Model file for the job. Use its own axes, mm. Face numbers are marked on the shaded views. A direction names the side the tool comes from. Coordinates: 2 decimals unless noted, no trailing zeros. Order: outer loops, then holes, each group sorted by start corner. A loop starts at its lowest first (then second) coordinate and runs counter-clockwise, first axis right, second up. Notation, with made-up numbers: (-30.5, 41) -> (7.5, 41) arc R29 ccw to (7.5, 74) -> close; hole circle Ø6 at (9, -8). An arc over 180 degrees is marked (long way). Use CSV: the item, a comma, the result in double quotes. Start each with the question number.
(1) Cut at B-B on x = 27.85. Write the cut outline in (y, z).
(2) Cut at A-A on z = 0. Write the cut outline in (x, y).
(3) Tool access for the marked faces 4, 5 and 6: list every direction of +Z, -Z, +X, -X, +Y, -Y with a clear straight run to the whole face (end or side of a thin tool).
(4) Pin check, flat tips, straight feed: pin 1 Ø3 at (y, z) = (2.5, 1.5) entering from +X; pin 2 Ø1.2 at (y, z) = (3, -11) entering from -X; pin 3 Ø4.5 at (x, z) = (13, -13) entering from +Y; pin 4 Ø8.5 at (x, y) = (27.85, -14) entering from -Z. Stop position of each tip, or through.
(5) Cut at C-C on x = 0. Write the cut outline in (y, z).
(6) Cut at D-D on y = -22. Write the cut outline in (x, z).
(7) Pull direction Z, two halves, no side cores. Call the marked faces 1, 2 and 3: pulls with the +Z half, pulls with the -Z half, needs draft (parallel to the pull), parting line crosses it, or undercut.
(8) Probe L1, parallel to X at y = 2, z = -13; L2, parallel to Z at x = 6.5, y = -8; L3, parallel to Z at x = 16.5, y = -1. List the from-to ranges inside material, lowest first.
Autodesk Inventor part; units mm, degrees
ref_plane "YZ Plane" through (0, 0, 0) normal (1, 0, 0) x (0, 1, 0)
ref_plane "XZ Plane" through (0, 0, 0) normal (0, 1, 0) x (-1, 0, 0)
ref_plane "XY Plane" through (0, 0, 0) normal (0, 0, 1) x (1, 0, 0)
sketch "Boceto1" plane through (0, 0, 0) normal (0, 1, 0) x (-1, 0, 0)
  line L0 (-17.55, 17.55) -> (17.55, 17.55)
  line L1 (17.55, 17.55) -> (17.55, -17.55)
  line L2 (17.55, -17.55) -> (-17.55, -17.55)
  line L3 (-17.55, -17.55) -> (-17.55, 17.55)
  line L4 (-17.55, 17.55) -> (17.55, -17.55) construction
  line L5 (17.55, 17.55) -> (-17.55, -17.55) construction
  circle A0 centre (0, 0) radius 11.2
  point P0 (0, 0)
  dimension "d0" = 35.1
  dimension "d1" = 35.1
  dimension "d2" = 22.4
extrude "Extrusión1" add sketch "Boceto1" along normal blind 4
sketch "Boceto2" plane through (0, 4, 0) normal (0, 1, 0) x (1, 0, 0)
  circle A0 centre (-13, -13) radius 1.7
  line L0 (13, -13) -> (-13, -13)
  line L1 (-13, -13) -> (-13, 13)
  line L2 (-13, 13) -> (13, 13)
  line L3 (13, 13) -> (13, -13)
  line L4 (13, -13) -> (-13, 13) construction
  line L5 (-13, -13) -> (13, 13) construction
  point P0 (0, 0)
  dimension "d5" = 26
  dimension "d6" = 26
  dimension "d7" = 3.4
extrude "Extrusión2" cut sketch "Boceto2" against normal through all contours L0 L1 A0 | A0 L1 L0
pattern_circular "Patrón circular1" count 4 over 360 about axis through (0, 0, 0) along (0, 1, 0) of "Extrusión2"
sketch "Boceto13" plane through (0, 4, 0) normal (0, 1, 0) x (1, 0, 0)
  line L0 (-17.55, -17.55) -> (17.55, -17.55)
  line L1 (17.55, -17.55) -> (37.85, -17.55)
  line L2 (37.85, -17.55) -> (37.85, 17.55)
  line L3 (37.85, 17.55) -> (17.55, 17.55)
  line L4 (17.55, 17.55) -> (17.55, -17.55)
  line L5 (17.55, 17.55) -> (-17.55, 17.55)
  line L6 (41.5, -10.15) -> (21.2, -10.15)
  line L7 (21.2, -10.15) -> (21.2, 10.15)
  line L8 (21.2, 10.15) -> (41.5, 10.15)
  line L9 (41.5, 10.15) -> (41.5, -10.15)
  line L10 (41.5, -10.15) -> (21.2, 10.15) construction
  line L11 (21.2, -10.15) -> (41.5, 10.15) construction
  circle A0 centre (27.85, 0) radius 2.7
  point P0 (0, 0)
  point P1 (31.35, 0)
  dimension "d43" = 20.3
  dimension "d44" = 20.3
  dimension "d45" = 20.3
  dimension "d61" = 5.4
  dimension "d62" = 10
extrude "Extrusión8" add sketch "Boceto13" against normal blind 33 contours L4 L3 L2 L8 L7 L6 L1 | L6 L7 L8 L2
sketch "Boceto14" plane through (0, -29, 0) normal (0, -1, 0) x (1, 0, 0)
  line L0 (17.55, 17.55) -> (17.55, -17.55)
  line L1 (37.85, -10.15) -> (17.55, -10.15)
  line L2 (17.55, -10.15) -> (17.55, 10.15)
  line L3 (17.55, 10.15) -> (37.85, 10.15)
  line L4 (37.85, 10.15) -> (37.85, -10.15)
  line L5 (37.85, -10.15) -> (17.55, 10.15) construction
  line L6 (17.55, -10.15) -> (37.85, 10.15) construction
  line L7 (37.85, -17.55) -> (37.85, 17.55)
  circle A0 centre (27.85, 0) radius 2.7
  point P0 (0, 0)
  point P1 (27.7, 0)
  point P2 (17.55, -10.15)
  point P3 (27.7, 0)
  dimension "d49" = 20.3
extrude "Extrusión9" cut sketch "Boceto14" against normal up to surface (29 mm away) contours L3 L4 L1 L0 | A0
sketch "Boceto15" plane through (-17.55, 0, -17.55) normal (0, 0, -1) x (-1, 0, 0)
  line L0 (-35.1, 0) -> (0, 0)
  line L1 (0, 0) -> (0, 4)
  line L2 (-55.4, 4) -> (0, 4)
  line L3 (-55.4, 4) -> (-55.4, -29)
  line L4 (-35.1, -29) -> (-55.4, -29)
  line L5 (-35.1, 0) -> (-35.1, -29)
  line L6 (0, 0) -> (0, 4)
  line L7 (-35.1, -29) -> (-55.4, -29)
  line L8 (0, 0) -> (-35.1, -29)
  point P0 (-17.55, 0)
extrude "Extrusión10" add sketch "Boceto15" along normal blind 2
mirror "Simetría1" about plane through (0, 0, 0) normal (0, 0, 1) of "Extrusión10"
sketch "Boceto16" plane through (-17.55, 0, -19.55) normal (0, 0, -1) x (-1, 0, 0)
  circle A0 centre (-45.4, -14) radius 2.7
  line L0 (-55.4, 4) -> (-55.4, -29)
  line L1 (-55.4, -29) -> (-35.1, -29)
  point P0 (-17.55, 0)
  dimension "d54" = 10
  dimension "d55" = 5.4
  dimension "d57" = 15
extrude "Extrusión11" cut sketch "Boceto16" against normal through all
fillet "Empalme1" radius 2 1 edges at (37.85, -29, -14.85)
sketch "Boceto17" plane through (-17.55, 0, -19.55) normal (0, 0, -1) x (-1, 0, 0)
  circle A0 centre (-45.4, -14) radius 2.7
  circle A1 centre (-45.4, -14) radius 4.65
  point P0 (-17.55, 0)
  dimension "d63" = 9.3
extrude "Extrusión12" cut sketch "Boceto17" against normal blind 2 contours A0 | A1
sketch "Boceto18" plane through (0, 4, 0) normal (0, 1, 0) x (1, 0, 0)
  circle A0 centre (27.85, 0) radius 2.7
  circle A1 centre (27.85, 0) radius 4.6
  point P0 (0, 0)
  dimension "d66" = 9.2
extrude "Extrusión13" cut sketch "Boceto18" against normal blind 2 contours A0 | A1
mirror "Simetría2" about plane through (0, 0, 0) normal (0, 0, 1) of "Extrusión12"
sketch "Boceto19" plane through (0, 4, 0) normal (0, 1, 0) x (1, 0, 0)
  line L0 (17.55, -17.55) -> (-17.55, -17.55)
  line L1 (-17.55, 17.55) -> (-17.55, -17.55)
  line L2 (-17.55, -17.55) -> (37.85, -17.55)
  line L3 (37.85, -17.55) -> (37.85, -39.55)
  line L4 (37.85, -39.55) -> (-17.55, -39.55)
  line L5 (-17.55, -39.55) -> (-17.55, -17.55)
  line L6 (-17.55, -19.55) -> (37.85, -19.55)
  line L7 (37.85, -19.55) -> (37.85, 19.55)
  line L8 (-17.55, -17.55) -> (-17.55, -19.55)
  line L9 (-17.55, -17.55) -> (-27.55, -17.55)
  line L10 (-27.55, -17.55) -> (-27.55, -39.55)
  line L11 (-27.55, -39.55) -> (-17.55, -39.55)
  line L12 (-17.55, -39.55) -> (-17.55, -17.55)
  point P0 (0, 0)
  dimension "d69" = 20
  dimension "d86" = 10
extrude "Extrusión14" add sketch "Boceto19" against normal blind 6
sketch "Boceto20" plane through (0, -2, 0) normal (0, -1, 0) x (1, 0, 0)
  circle A0 centre (-18.875, 33.55) radius 2.7
  circle A1 centre (14.55, 33.55) radius 2.7
  line L0 (37.85, 19.55) -> (37.85, 39.55)
  line L1 (-27.55, 39.55) -> (-27.55, 17.55)
  line L2 (37.85, 39.55) -> (-27.55, 39.55)
  point P0 (0, 0)
  dimension "d72" = 5.4
  dimension "d74" = 23.3
  dimension "d87" = 8.675
  dimension "d88" = 6
extrude "Extrusión15" cut sketch "Boceto20" against normal through all
sketch "Boceto21" plane through (0, -2, 0) normal (0, -1, 0) x (1, 0, 0)
  circle A0 centre (-18.875, 33.55) radius 2.7
  circle A1 centre (-18.875, 33.55) radius 4.05
  circle A2 centre (14.55, 33.55) radius 2.7
  circle A3 centre (14.55, 33.55) radius 4.05
  line L0 (14.55, 38.2265) -> (18.6, 35.8883)
  line L1 (18.6, 35.8883) -> (18.6, 31.2117)
  line L2 (18.6, 31.2117) -> (14.55, 28.8735)
  line L3 (14.55, 28.8735) -> (10.5, 31.2117)
  line L4 (10.5, 31.2117) -> (10.5, 35.8883)
  line L5 (10.5, 35.8883) -> (14.55, 38.2265)
  line L6 (-18.875, 38.2265) -> (-14.825, 35.8883)
  line L7 (-14.825, 35.8883) -> (-14.825, 31.2117)
  line L8 (-14.825, 31.2117) -> (-18.875, 28.8735)
  line L9 (-18.875, 28.8735) -> (-22.925, 31.2117)
  line L10 (-22.925, 31.2117) -> (-22.925, 35.8883)
  line L11 (-22.925, 35.8883) -> (-18.875, 38.2265)
  point P0 (0, 0)
  dimension "d79" = 8.1
extrude "Extrusión16" cut sketch "Boceto21" against normal blind 4 contours A0 | A1 | L7 L8 A1 | A1 L6 L7 | A1 L11 L6 | L8 L9 A1 | A1 L10 L11 | L9 L10 A1 | A2 | A3 | L1 L2 A3 | A3 L0 L1 | A3 L5 L0 | L2 L3 A3 | A3 L4 L5 | L3 L4 A3
fillet "Empalme2" radius 3 1 edges at (37.85, 1, 39.55)
fillet "Empalme3" radius 5 1 edges at (11.3603, -2, 19.55)
sketch "Boceto22" plane through (0, 4, 0) normal (0, 1, 0) x (1, 0, 0)
  line L0 (37.85, -10.15) -> (37.85, 10.15)
  line L1 (35.85, 10.15) -> (17.55, 10.15)
  line L2 (37.85, -10.15) -> (17.55, -10.15)
  line L3 (17.55, -10.15) -> (17.55, 10.15)
  line L4 (17.55, 10.15) -> (37.85, 10.15)
  line L5 (37.85, 10.15) -> (37.85, -10.15)
  line L6 (17.55, 10.15) -> (17.55, 17.55)
  point P0 (0, 0)
extrude "Extrusión17" cut sketch "Boceto22" against normal through all
fillet "Empalme4" radius 5 3 edges at (-27.55, 1, 39.55) (-27.55, 1, 17.55) (-17.55, 2, 17.55)
sketch "Boceto24" plane through (0, -2, 0) normal (0, -1, 0) x (1, 0, 0)
  point P0 (0, 0)
sketch "Boceto7" plane through (17.55, 0, -17.55) normal (0, 0, -1) x (-1, 0, 0)
  line L0 (35.1, 0) -> (35.1, 4)
  line L1 (35.1, 4) -> (-20.3, 4)
  line L2 (-20.3, 4) -> (-20.3, -26)
  line L3 (-20.3, -26) -> (35.1, -26)
  line L4 (35.1, -26) -> (35.1, 4)
  line L5 (0, 0) -> (0, 4)
  point P0 (17.55, 0)
  point P1 (35.6, 0)
  dimension "d23" = 20.3
  dimension "d24" = 30
sketch "Boceto8" plane through (0, 3, 0) normal (0, 1, 0) x (1, 0, 0)
  line L0 (17.8, 17.8) -> (-17.8, 17.8)
  line L1 (17.8, -17.8) -> (16.8, -17.8)
  line L2 (16.8, -17.8) -> (16.8, 17.8)
  line L3 (16.8, 17.8) -> (17.8, 17.8)
  line L4 (17.8, 17.8) -> (17.8, -17.8)
  point P0 (0, 0)
  dimension "d27" = 1
sketch "Boceto9" plane through (17.8, 0, -21.8) normal (0, 0, -1) x (-1, 0, 0)
  circle A0 centre (-10.3, -4.5) radius 2.7
  circle A1 centre (-10.3, -19.5) radius 2.7
  line L0 (-20.3, 3) -> (-20.3, -27)
  line L1 (35.6, 3) -> (-20.3, 3)
  line L2 (-20.3, -27) -> (35.6, -27)
  point P0 (17.8, 0)
  dimension "d30" = 5.4
  dimension "d31" = 10
  dimension "d32" = 7.5
  dimension "d33" = 7.5
  dimension "d41" = 80
  dimension "d42" = 20.3
sketch "Boceto10" plane through (17.8, 0, -17.8) normal (0, 0, 1) x (1, 0, 0)
  line L0 (20.3, 3) -> (20.3, -27)
  line L1 (-1, 3) -> (20.3, 3)
  line L2 (20.3, -27) -> (0.3, -27)
  line L3 (0.3, -27) -> (0.3, 3)
  line L4 (0.3, 3) -> (20.3, 3)
  line L5 (20.3, 3) -> (20.3, -27)
  circle A0 centre (10.3, -4.5) radius 2.7
  circle A1 centre (10.3, -19.5) radius 2.7
  line L6 (-1, 0) -> (-35.6, 0)
  line L7 (-35.6, -27) -> (-35.6, 0)
  line L8 (20.3, -27) -> (-35.6, -27)
  line L9 (20.3, 3) -> (20.3, -27)
  line L10 (-1, 3) -> (20.3, 3)
  line L11 (-1, 3) -> (-1, 0)
  point P0 (-17.8, 0)
  dimension "d36" = 20
sketch "Boceto3" plane through (-17.55, 0, 17.55) normal (0, 0, 1) x (1, 0, 0)
  line L0 (0, 0) -> (0, 4)
  line L1 (0, 4) -> (55.4, 4)
  line L2 (55.4, 4) -> (55.4, -30)
  line L3 (55.4, -30) -> (0, -30)
  line L4 (0, -30) -> (0, 4)
  line L5 (35.1, 0) -> (35.1, 4)
  line L6 (0, 0) -> (35.1, 0)
  point P0 (17.55, 0)
  dimension "d13" = 20.3
  dimension "d14" = 30
  dimension "d17" = 5.4
  dimension "d18" = 10
  dimension "d19" = 7.5
  dimension "d20" = 7.5
  dimension "d21" = 20.3
  dimension "d22" = 20.3
properties part number "NEMA14 support"
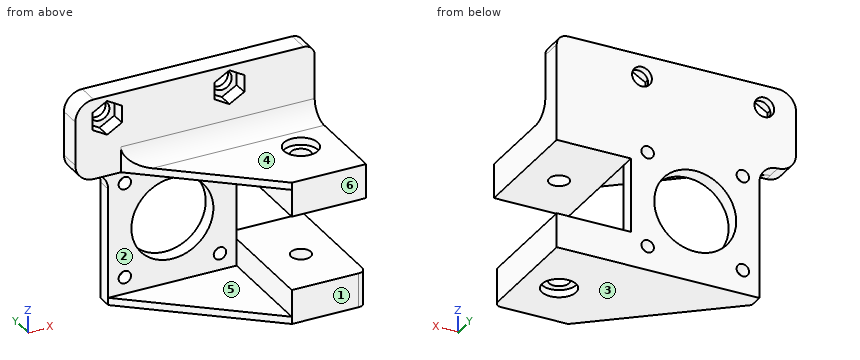
Outcome:
1,outline,"(-29, -19.55) -> (-18.65, -19.55) -> (-18.65, -17.55) -> (-16.7, -17.55) -> (-16.7, -10.15) -> (-29, -10.15) -> close; (-29, 10.15) -> (-16.7, 10.15) -> (-16.7, 17.55) -> (-18.65, 17.55) -> (-18.65, 19.55) -> (-29, 19.55) -> close; (-11.3, -17.55) -> (-9.35, -17.55) -> (-9.35, -19.55) -> (4, -19.55) -> (4, -10.15) -> (-11.3, -10.15) -> close; (-11.3, 10.15) -> (4, 10.15) -> (4, 39.55) -> (-2, 39.55) -> (-2, 24.55) arc R5 cw to (-7, 19.55) -> (-9.35, 19.55) -> (-9.35, 17.55) -> (-11.3, 17.55) -> close"
2,outline,"(-17.55, 0) -> (-11.2, 0) -> (-11.2, 4) -> (-17.55, 4) -> close; (11.2, 0) -> (17.55, 0) -> (17.55, 4) -> (11.2, 4) -> close"
3,face 4,"+Z, +X, -X, -Y"
3,face 5,"-X, -Y"
3,face 6,"+Z, -Z, +X, -X, -Y"
4,pin 1,"x = 17.55"
4,pin 2,"x = -17.55"
4,pin 3,"y = 4"
4,pin 4,"z = -17.55"
5,outline,"(-14.5, -19.55) -> (4, -19.55) -> (4, -11.2) -> (0, -11.2) -> (0, -17.55) -> (-14.5, -17.55) -> close; (-14.5, 17.55) -> (0, 17.55) -> (0, 11.2) -> (4, 11.2) -> (4, 39.55) -> (-2, 39.55) -> (-2, 24.55) arc R5 cw to (-7, 19.55) -> (-14.5, 19.55) -> close"
6,outline,"(9.08, -19.55) -> (37.85, -19.55) -> (37.85, -10.15) -> (17.55, -10.15) -> (17.55, -17.55) -> (9.08, -17.55) -> close; (9.08, 17.55) -> (17.55, 17.55) -> (17.55, 10.15) -> (37.85, 10.15) -> (37.85, 19.55) -> (9.08, 19.55) -> close"
7,face 1,"needs draft"
7,face 2,"undercut"
7,face 3,"pulls with the -Z half"
8,L1,"-17.55 to -14.7, -11.3 to 11.3, 14.7 to 37.85"
8,L2,"-19.55 to -17.55, 17.55 to 19.55"
8,L3,"-19.55 to -17.55, 17.55 to 30, 37.1 to 39.55"
